from build123d import *

# Parameters (mm, degrees)
BOSS_EXTRUDE1_DEPTH = 10
CUT_EXTRUDE1_DEPTH  = 7
BOSS_EXTRUDE2_START = -50
BOSS_EXTRUDE2_DEPTH = 50
CUT_EXTRUDE2_DEPTH  = 40
CUT_EXTRUDE3_DEPTH  = 7


with BuildPart() as part:
    # Sketch1 → Boss-Extrude1 (new body)
    with BuildSketch(Plane(origin=(0, 157.279655443, 0), x_dir=(1, 0, 0), z_dir=(0, 1, 0))):
        with BuildLine():
            Line((293.03566289, -316.199227389), (265.928972249, -322.110427169))
            ThreePointArc((265.928972249, -322.110427169), (252.377607393, -287.084094578), (228.819595995, -257.835102061))
            Line((228.819595995, -257.835102061), (247.492190492, -237.315619243))
            ThreePointArc((247.492190492, -237.315619243), (255.674613952, -244.45932236), (263.205967645, -252.286407351))
            Line((263.205967645, -252.286407351), (248.454819921, -268.496576877))
            Line((248.454819921, -268.496576877), (257.330112784, -276.573035048))
            Line((257.330112784, -276.573035048), (270.790876402, -261.780880276))
            ThreePointArc((270.790876402, -261.780880276), (277.704929826, -272.461358153), (283.49746828, -283.789342999))
            Line((283.49746828, -283.789342999), (263.956704662, -288.050628861))
            Line((263.956704662, -288.050628861), (266.513476179, -299.775087033))
            Line((266.513476179, -299.775087033), (287.92746865, -295.105303131))
            ThreePointArc((287.92746865, -295.105303131), (290.940246243, -305.54118925), (293.03566289, -316.199227389))
        make_face()
    extrude(amount=BOSS_EXTRUDE1_DEPTH)

    # Sketch2 → Cut-Extrude1 (cut)
    with BuildSketch(Plane(origin=(0, 157.279655443, 0), x_dir=(1, 0, 0), z_dir=(0, 1, 0))):
        Polygon((267.822908947, -321.697413337), (265.266137429, -309.972955165), (295.554321038, -303.367962079), (297.930502387, -315.13180184), align=None)
        Polygon((251.029855966, -233.428046687), (230.165672357, -256.355886583), (239.04096522, -264.432344755), (259.905148829, -241.504504858), align=None)
    extrude(amount=CUT_EXTRUDE1_DEPTH, mode=Mode.SUBTRACT)

    # Sketch3 → Boss-Extrude2 (add)
    with BuildSketch(Plane(origin=(0, 167.279655443, 0), x_dir=(1, 0, 0), z_dir=(0, 1, 0)).offset(BOSS_EXTRUDE2_START)):
        with BuildLine():
            Line((293.03566289, -316.199227389), (298.897891976, -314.920841631))
            ThreePointArc((298.897891976, -314.920841631), (281.600541129, -270.212225919), (251.530419577, -232.877972811))
            Line((251.530419577, -232.877972811), (247.492190492, -237.315619243))
            ThreePointArc((247.492190492, -237.315619243), (277.704929826, -272.461358153), (293.03566289, -316.199227389))
        make_face()
    extrude(amount=BOSS_EXTRUDE2_DEPTH)

    # Sketch4 → Cut-Extrude2 (cut)
    with BuildSketch(Plane.XZ.offset(-117.279655443)):
        with BuildLine():
            Line((293.03566289, 316.199227389), (294.012701071, 315.986163096))
            ThreePointArc((294.012701071, 315.986163096), (278.53244595, 271.983591496), (248.165228673, 236.576011504))
            Line((248.165228673, 236.576011504), (247.492190492, 237.315619243))
            ThreePointArc((247.492190492, 237.315619243), (277.704929826, 272.461358153), (293.03566289, 316.199227389))
        make_face()
    extrude(amount=-CUT_EXTRUDE2_DEPTH, mode=Mode.SUBTRACT)

    # Sketch5 → Cut-Extrude3 (cut)
    with BuildSketch(Plane(origin=(0, 157.279655443, 0), x_dir=(1, 0, 0), z_dir=(0, 1, 0))):
        Polygon((249.934035398, -269.842653239), (255.850897307, -275.226958686), (249.120515497, -282.623036072), (243.203653588, -277.238730625), align=None)
        Polygon((264.382833248, -290.004705223), (266.087347593, -297.821010671), (256.316965783, -299.951653602), (254.612451439, -292.135348154), align=None)
    extrude(amount=CUT_EXTRUDE3_DEPTH, mode=Mode.SUBTRACT)


solid = part.part
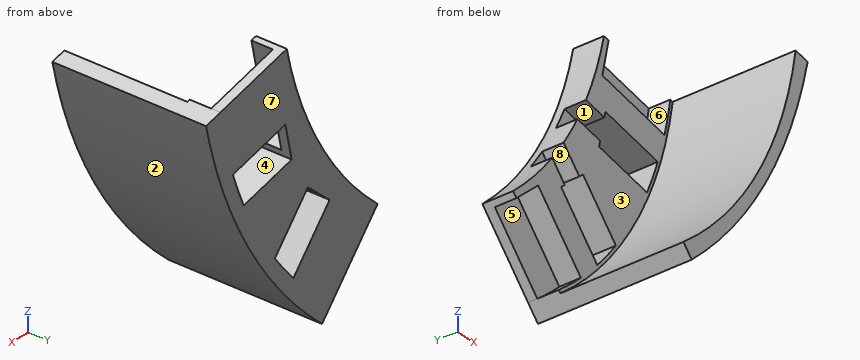
For this review, take the finished solid that the model builds, in its own axes (mm). Face numbers are marked on the shaded views. A direction names the side the tool comes from. Round coordinates to 2 decimals unless told otherwise and drop trailing zeros. Order: outer loops, then holes, each group sorted by start corner. A loop starts at its lowest first (then second) coordinate and runs counter-clockwise, first axis right, second up. Notation, with made-up numbers: M 31.25,83.25 L 61.25,83.25 A18 ccw 61.25,115.25 Z; hole C 30.5,-3.5 d7. An arc over 180 degrees is marked long. Write each question's results on one line, items separated by ' | '. Start each with the question number.
1. Add section A-A (z = 271). State the section outline as (x, y) points, then the cut area to 3 significant figures.
2. Draft analysis for pull direction Z (two halves, no side actions). For the marked faces 6, 7 and 8, state which applies: pulls with the +Z half, pulls with the -Z half, needs draft (parallel to the pull), parting line crosses it, or undercut.
3. Clearance check with flat-ended pins moving along their axes: pin 1 Ø7.5 at (x, z) = (262, 294) entering from -Y; pin 2 Ø4 at (y, z) = (125.5, 302.5) entering from +X; pin 3 Ø8 at (x, z) = (250, 245) entering from -Y. State where each tip first meets the part, or that it passes through.
4. Tool access review of the marked faces 1, 2, 3, 4 and 5: name each direction out of +Z, -Z, +X, -X, +Y, -Y from which nothing blocks a thin tool from reaching the whole face with its end or side.
5. Add section C-C (y = 159). State the section outline as (x, z) points, then the cut area to 3 significant figures.
6. Add section D-D (x = 241). State the section outline as (y, z) points, then the cut area to 3 significant figures.
7. Add section B-B (x = 274). State the section outline as (y, z) points, then the cut area to 3 significant figures.
8. To check wall thickness, follow L1, parallel to Z at x = 270.5, y = 165.5; L2, parallel to Y at x = 246.5, z = 244; L3, parallel to Y at x = 279, z = 277.5. State the ranges of each line that lie inside material, in increasing order. Write a range as [from, to].
Output values:
1) outline: M 241.29,157.28 L 248.88,157.28 L 248.88,164.28 L 251.21,164.28 L 251.21,167.28 L 241.29,167.28 Z; M 262.4,157.28 L 277.96,157.28 L 277.96,117.28 L 282.05,117.28 L 282.05,167.28 L 262.4,167.28 Z | area: 443 mm^2
2) face 6: pulls with the +Z half | face 7: needs draft | face 8: undercut
3) pin 1: y = 157.28 | pin 2: x = 296.25 | pin 3: y = 164.28
4) face 1: -X, -Y | face 2: -Z, +X, +Y, -Y | face 3: +Z, -X, -Y | face 4: +Y, -Y | face 5: -Y
5) outline: M 228.82,257.84 L 230.17,256.36 L 239.04,264.43 L 256.5,245.25 A125 cw 247.49,237.32 L 251.53,232.88 A155.81 ccw 298.9,314.92 L 293.04,316.2 A125 cw 290.67,304.43 L 265.27,309.97 L 267.82,321.7 L 265.93,322.11 A122.07 cw 258.61,299.45 L 266.09,297.82 L 266.51,299.78 L 287.93,295.11 A125 cw 283.5,283.79 L 263.96,288.05 L 264.38,290 L 255.08,292.03 A122.07 cw 249.45,282.27 L 255.85,275.23 L 257.33,276.57 L 270.79,261.78 A125 cw 263.21,252.29 L 248.45,268.5 L 249.93,269.84 L 244.78,275.5 A122.07 cw Z | area: 1,630 mm^2
6) outline: M 157.28,262.28 L 164.28,262.28 L 164.28,244.45 L 167.28,244.45 L 167.28,270.65 L 157.28,270.65 Z | area: 137 mm^2
7) outline: M 117.28,258.33 L 167.28,258.33 L 167.28,285.86 L 157.28,285.86 L 157.28,264.71 L 117.28,264.71 Z; M 157.28,298.14 L 167.28,298.14 L 167.28,320.35 L 164.28,320.35 L 164.28,308.07 L 157.28,308.07 Z | area: 667 mm^2
8) L1: [253.56, 261.38], [262.1, 286.62], [298.91, 321.11] | L2: [164.28, 167.28] | L3: [157.28, 167.28]
